from build123d import *

# Parameters (mm, degrees)
SKETCH_1_W          = 20
SKETCH_1_H          = 13
EXTRUDE_1_DEPTH     = 12
SHELL_1_T           = -1
SKETCH_2_R          = 2.5
SKETCH_2_R_2        = 2
EXTRUDE_4_DEPTH     = 10
SKETCH_3_R          = 4.9
CUT_EXTRUDE_1_DEPTH = 0.2
SKETCH_9_R          = 2.5
SKETCH_9_R_2        = 2
EXTRUDE_8_DEPTH     = 10
SKETCH_6_W          = 2
SKETCH_6_H          = 10
EXTRUDE_10_DEPTH    = 3
SKETCH_10_W         = 2
SKETCH_10_H         = 10
EXTRUDE_11_DEPTH    = 3
SCALE_1_SCALE       = 2


with BuildPart() as part:
    # Sketch 1 → Extrude 1 (new body)
    with BuildSketch(Plane.XY):
        Rectangle(SKETCH_1_W, SKETCH_1_H)
    extrude(amount=EXTRUDE_1_DEPTH)

    # Shell 1
    shell_1_openings = [part.faces().sort_by_distance(p)[0] for p in [
        (0, 0, 12),
    ]]
    offset(amount=SHELL_1_T, openings=shell_1_openings, kind=Kind.INTERSECTION)

    # Sketch 3 → Cut-Extrude 1 (cut)
    with BuildSketch(Plane.XY.offset(1)):
        Circle(SKETCH_3_R)
    extrude(amount=-CUT_EXTRUDE_1_DEPTH, mode=Mode.SUBTRACT)

    # Sketch 9 → Extrude 8 (add)
    # profile 1 of 3: a face of its own
    with BuildSketch(Plane(origin=(0, 6.5, 0), x_dir=(1, 0, 0), z_dir=(0, 1, 0))):
        with BuildLine():
            Line((10, -14.5), (10, -12))
            Line((10, -12), (7.5, -12))
            ThreePointArc((7.5, -12), (9.267766953, -12.732233047), (10, -14.5))
        make_face()
    # profile 2 of 3: a face of its own
    with BuildSketch(Plane(origin=(0, 6.5, 0), x_dir=(1, 0, 0), z_dir=(0, 1, 0))):
        with BuildLine():
            Line((10, -17), (10, -14.5))
            ThreePointArc((10, -14.5), (9.267766953, -16.267766953), (7.5, -17))
            Line((7.5, -17), (10, -17))
        make_face()
    # profile 3 of 3: a face of its own
    with BuildSketch(Plane(origin=(0, 6.5, 0), x_dir=(1, 0, 0), z_dir=(0, 1, 0))):
        with Locations((7.5, -14.5)):
            Circle(SKETCH_9_R)
        with Locations(Location((7.5, -14.5, 0), (0, 0, 270))):
            Circle(SKETCH_9_R_2, mode=Mode.SUBTRACT)
    extrude(amount=-EXTRUDE_8_DEPTH)


with BuildPart() as body_2:
    # Sketch 2 → Extrude 4 (new body)
    # profile 1 of 3: a face of its own
    with BuildSketch(Plane(origin=(0, 3.5, 0), x_dir=(1, 0, 0), z_dir=(0, 1, 0))):
        with BuildLine():
            ThreePointArc((-7.5, -17), (-9.267766953, -16.267766953), (-10, -14.5))
            Line((-10, -14.5), (-10, -17))
            Line((-10, -17), (-7.5, -17))
        make_face()
    # profile 2 of 3: a face of its own
    with BuildSketch(Plane(origin=(0, 3.5, 0), x_dir=(1, 0, 0), z_dir=(0, 1, 0))):
        with Locations((-7.5, -14.5)):
            Circle(SKETCH_2_R)
        with Locations(Location((-7.5, -14.5, 0), (0, 0, 270))):
            Circle(SKETCH_2_R_2, mode=Mode.SUBTRACT)
    # profile 3 of 3: a face of its own
    with BuildSketch(Plane(origin=(0, 3.5, 0), x_dir=(1, 0, 0), z_dir=(0, 1, 0))):
        with BuildLine():
            Line((-7.5, -12), (-10, -12))
            Line((-10, -12), (-10, -14.5))
            ThreePointArc((-10, -14.5), (-9.267766953, -12.732233047), (-7.5, -12))
        make_face()
    extrude(amount=-EXTRUDE_4_DEPTH)


    add(part.part)  # Extrude 10 merges part
    # Sketch 6 → Extrude 10 (add)
    with BuildSketch(Plane.ZY.offset(10)):
        with Locations((16, -1.5)):
            Rectangle(SKETCH_6_W, SKETCH_6_H)
    extrude(amount=EXTRUDE_10_DEPTH)

    # Sketch 10 → Extrude 11 (add)
    with BuildSketch(Plane(origin=(10, 0, 0), x_dir=(0, 0, -1), z_dir=(1, 0, 0))):
        with Locations((-16, 1.5)):
            Rectangle(SKETCH_10_W, SKETCH_10_H)
    extrude(amount=EXTRUDE_11_DEPTH)


with BuildPart() as body_2_1:
    # Scale 1: scaled about (0, 0, 0)
    add(body_2.part.scale(SCALE_1_SCALE))


solid = body_2_1.part
Geometry check sheet. Reference: the model listing, model coordinates, mm. A direction names the side the tool comes from. Round coordinates to 2 decimals unless told otherwise and drop trailing zeros. Order: outer loops, then holes, each group sorted by start corner. A loop starts at its lowest first (then second) coordinate and runs counter-clockwise, first axis right, second up. Notation, with made-up numbers: (66.25, 31) - (102.25, 31) arc R20 cw to (102.25, 47) - close; hole circle Ø11 at (59.5, 80). An arc over 180 degrees is marked (long way). One line per question, with ' | ' between items. Start each with the question number.
(1) Sectioned sample at D-D on x = -12. Record the cut outline in (y, z).
(2) Thickness scan on L1, parallel to X at y = 3.25, z = 29; L2, parallel to Y at x = 9.5, z = 20; L3, parallel to X at y = -9.5, z = 22.5. Record the ranges inside material, lowest first. Write a range as [from, to].
(3) Sectioned sample at B-B on y = 0. Record the cut outline in (x, z), and give its area (3 significant figures).
(4) Access from +Z, -Z, +X, -X, +Y, -Y to the whole of each face (thin tool, end or side, straight path). Record for faces 5 (the flat face through (0, -11, 13)), 6 (the cylindrical face through (-2.124, -9.567, 1.803)), 7 (the flat face through (-23, -3, 30)).
(5) Sectioned sample at A-A on z = 14. Record the cut outline in (x, y).
(6) Release check for a two-part mould opening along Z. For faces 1 (the cylindrical face through (-12.3, -2.86, 26.05)), 2 (the flat face through (23, 3, 30)), 3 (the flat face through (19.7, -7, 30.2)), 4 (the flat face through (0, 0, 1.6)) record: released by +Z, released by -Z, zero draft, split by the parting line, or undercut.
(7) Depth check by flat-ended pin: pin 1 Ø1.8 at (x, y) = (22, 6.5) entering from -Z; pin 2 Ø13 at (y, z) = (-6.5, 17.5) entering from -X; pin 3 Ø2.5 at (x, y) = (17, 1) entering from -Z; pin 4 Ø6 at (x, y) = (3, 2) entering from +Z. Enter the tip coordinate at first touch or a pass-through.
(8) Sectioned sample at C-C on z = 27. Record the cut outline in (x, y).
Conclusion:
1) outline: (-13, 0) - (13, 0) - (13, 24) - (11, 24) - (11, 2) - (-11, 2) - (-11, 24) - (-13, 24) - close; (-13, 25) - (7, 25) - (7, 26.35) - (-13, 26.35) - close; (-13, 31.65) - (7, 31.65) - (7, 33) - (-13, 33) - close
2) L1: x = [-20, -19], [-11, -10], [10, 11], [19, 20] | L2: y = [-13, -11], [11, 13] | L3: x = [-20, -18], [18, 20]
3) outline: (-26, 30) - (-20, 30) - (-20, 0) - (20, 0) - (20, 30) - (26, 30) - (26, 34) - (15, 34) arc R5 ccw to (15, 24) - (18, 24) - (18, 2) - (9.8, 2) - (9.8, 1.6) - (-9.8, 1.6) - (-9.8, 2) - (-18, 2) - (-18, 24) - (-15, 24) arc R5 ccw to (-15, 34) - (-26, 34) - close; hole circle Ø8 at (-15, 29); hole circle Ø8 at (15, 29) | area: 286 mm2
4) face 5: none | face 6: +Z | face 7: -Z, -X, +Y, -Y
5) outline: (-20, -13) - (20, -13) - (20, 13) - (-20, 13) - close; hole (-18, -11) - (18, -11) - (18, 11) - (-18, 11) - close
6) face 1: undercut | face 2: released by -Z | face 3: zero draft | face 4: released by +Z
7) pin 1: stops at z = 30 | pin 2: stops at x = -20 | pin 3: stops at z = 0 | pin 4: stops at z = 1.6
8) outline: (-20, -13) - (-18.46, -13) - (-18.46, 7) - (-20, 7) - close; (-11.54, -13) - (-10.42, -13) - (-10.42, 7) - (-11.54, 7) - close; (10.42, -7) - (11.54, -7) - (11.54, 13) - (10.42, 13) - close; (18.46, -7) - (20, -7) - (20, 13) - (18.46, 13) - close
